from build123d import *

# Parameters (mm, degrees)
BOSS_EXTRU_1_DEPTH      = 3
ESQUISSE3_W             = 36
ESQUISSE3_H             = 12
ENL_V_MAT_EXTRU_1_DEPTH = 4
SKETCH1_R               = 1.6
CUT_EXTRUDE1_DEPTH      = 71.150285103
SKETCH2_R               = 1.6
CUT_EXTRUDE2_DEPTH      = 71.150285103
SKETCH3_R               = 1.6
CUT_EXTRUDE3_DEPTH      = 71.150285103


with BuildPart() as part:
    # Esquisse1 → Boss.-Extru.1 (new body)
    with BuildSketch(Plane.XY):
        Polygon((61.25, -25), (-61.25, -25), (-61.25, -12.5), (-64.25, -12.5), (-64.25, 12.5), (-61.25, 12.5), (-61.25, 25), (-29.85, 25), (-26.65, 25), (-12.5, 25), (-12.5, 28), (12.5, 28), (12.5, 25), (26.65, 25), (29.85, 25), (61.25, 25), (61.25, 12.5), (64.25, 12.5), (64.25, -12.5), (61.25, -12.5), align=None)
    extrude(amount=BOSS_EXTRU_1_DEPTH)

    # Esquisse3 → Enlèv. mat.-Extru.1 (cut)
    with BuildSketch(Plane(origin=(0, 0, 0), x_dir=(-1, 0, 0), z_dir=(0, 0, -1))):
        with Locations((-0.047688523, 17.043645632)):
            Rectangle(ESQUISSE3_W, ESQUISSE3_H)
    extrude(amount=-ENL_V_MAT_EXTRU_1_DEPTH, mode=Mode.SUBTRACT)

    # Sketch1 → Cut-Extrude1 (cut, through all)
    with BuildSketch(Plane.XY.offset(3)):
        with Locations((35.25, 21)):
            Circle(SKETCH1_R)
    extrude(amount=-CUT_EXTRUDE1_DEPTH, mode=Mode.SUBTRACT)

    # Sketch2 → Cut-Extrude2 (cut, through all)
    with BuildSketch(Plane.XY.offset(3)):
        with Locations((-35.25, 21)):
            Circle(SKETCH2_R)
    extrude(amount=-CUT_EXTRUDE2_DEPTH, mode=Mode.SUBTRACT)

    # Sketch3 → Cut-Extrude3 (cut, through all)
    with BuildSketch(Plane.XY.offset(3)):
        with Locations((-35.25, -18.9)):
            Circle(SKETCH3_R)
        with Locations((35.25, -18.9)):
            Circle(SKETCH3_R)
    extrude(amount=-CUT_EXTRUDE3_DEPTH, mode=Mode.SUBTRACT)


solid = part.part
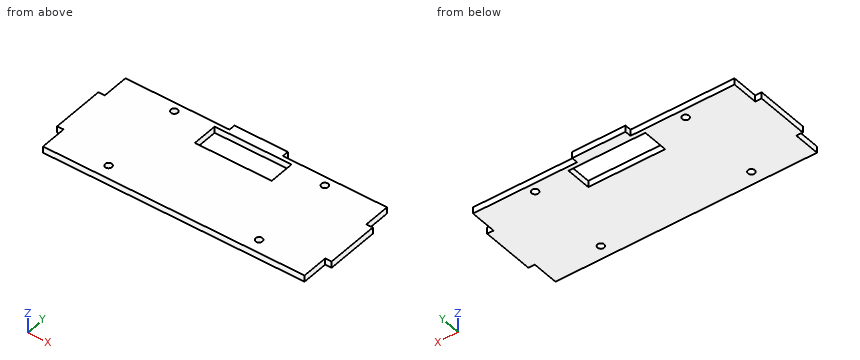
Here's how the part is built. I have some questions about the finished solid (model axes, mm). Round coordinates to 2 decimals unless told otherwise and drop trailing zeros. Write each loop counter-clockwise with the first axis right and the second up, starting at its lowest first coordinate (ties: lowest second). Pieces come first, ordered by that corner, then holes.
1. I need wall thicknesses on L1, parallel to Y at x = -35, z = 0.75; L2, parallel to Y at x = -7, z = 1.8; L3, parallel to Y at x = -16, z = 1.7. Which ranges of each line are inside material? Lowest first, please.
2. Suppose I cut it at D-D (z = 0.9). List the corners of the cut face in (x, y) for me.
3. Suppose I cut it at C-C (x = 15.5). List the corners of the cut face in (y, z) for me.
4. Suppose I cut it at B-B (y = 21). List the corners of the cut face in (x, z) for me.
5. Suppose I cut it at A-A (x = -35.25). List the corners of the cut face in (y, z) for me.
6. Will these pins go through, and if not, where does the flat tip stop? pin 1 Ø1.9 at (x, y) = (35.25, -18.9) entering from +Z; pin 2 Ø0.9 at (x, z) = (-62.5, 2) entering from -Y; pin 3 Ø0.9 at (y, z) = (18.5, 2) entering from +X; pin 4 Ø1.5 at (y, z) = (21.5, 1.5) entering from -X.
Answer sheet:
1. L1: y = -25 to -20.48, -17.32 to 19.42, 22.58 to 25
1. L2: y = -25 to 11.04, 23.04 to 28
1. L3: y = -25 to 11.04, 23.04 to 25
2. outline: (-64.25, -12.5) - (-61.25, -12.5) - (-61.25, -25) - (61.25, -25) - (61.25, -12.5) - (64.25, -12.5) - (64.25, 12.5) - (61.25, 12.5) - (61.25, 25) - (12.5, 25) - (12.5, 28) - (-12.5, 28) - (-12.5, 25) - (-61.25, 25) - (-61.25, 12.5) - (-64.25, 12.5) - close; hole circle Ø3.2 at (-35.25, -18.9); hole circle Ø3.2 at (-35.25, 21); hole (-17.95, 11.04) - (18.05, 11.04) - (18.05, 23.04) - (-17.95, 23.04) - close; hole circle Ø3.2 at (35.25, -18.9); hole circle Ø3.2 at (35.25, 21)
3. outline: (-25, 0) - (11.04, 0) - (11.04, 3) - (-25, 3) - close; (23.04, 0) - (25, 0) - (25, 3) - (23.04, 3) - close
4. outline: (-61.25, 0) - (-36.85, 0) - (-36.85, 3) - (-61.25, 3) - close; (-33.65, 0) - (-17.95, 0) - (-17.95, 3) - (-33.65, 3) - close; (18.05, 0) - (33.65, 0) - (33.65, 3) - (18.05, 3) - close; (36.85, 0) - (61.25, 0) - (61.25, 3) - (36.85, 3) - close
5. outline: (-25, 0) - (-20.5, 0) - (-20.5, 3) - (-25, 3) - close; (-17.3, 0) - (19.4, 0) - (19.4, 3) - (-17.3, 3) - close; (22.6, 0) - (25, 0) - (25, 3) - (22.6, 3) - close
6. pin 1: passes through
6. pin 2: stops at y = -12.5
6. pin 3: stops at x = 61.25
6. pin 4: stops at x = -61.25
